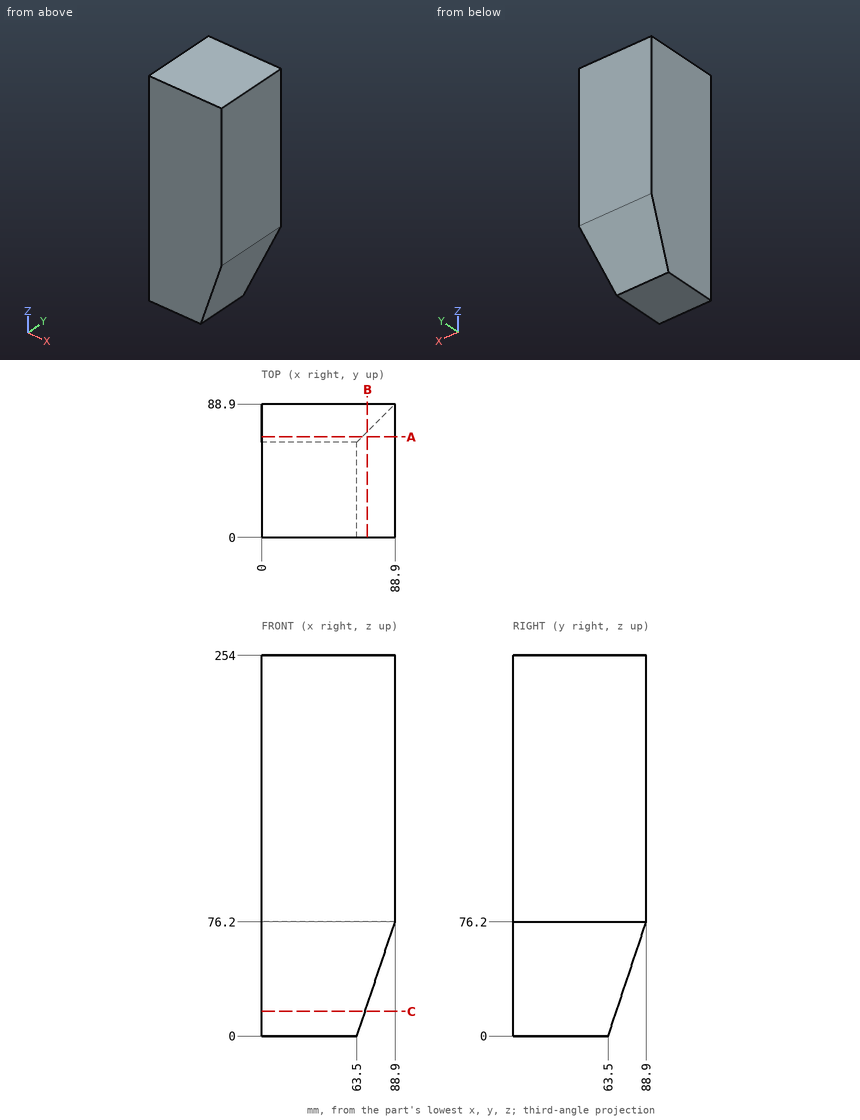
Here's the drawing with two shaded views (mm, measured from the low corner). I have some questions. Coordinates: 2 decimals unless noted, no trailing zeros. Loops run counter-clockwise (first coordinate to the right, second up) from the corner with the lowest first, then second, coordinate; pieces in that order, holes last. Notation, with made-up numbers: M -33,-34 L 4,-34 A19 ccw 4,-30 Z; hole C 86.25,-28.5 d2. An arc over 180 degrees is marked long. Put each result on its own line as item: value. Start each with the question number.
(1) Imagine slicing it at B-B on x = 70.5. List the corners of the cut face in (y, z) for me.
(2) I need wall thicknesses on probe 1 along X at (y, z) = (32.5, 61); probe 2 along X at (y, z) = (67.5, 36.5); probe 3 along Y at (x, z) = (66, 34.5). Which ranges of each line are inside material? Lowest first, please.
(3) Imagine slicing it at C-C on z = 16.5. List the corners of the cut face in (x, y) for me, and give its area (3 significant figures).
(4) Imagine slicing it at A-A on y = 67. List the corners of the cut face in (x, z) for me.
Worked answers:
1. outline: M 0,21 L 70.5,21 L 88.9,76.2 L 88.9,254 L 0,254 Z
2. probe 1: x = 0 to 83.83
2. probe 2: x = 0 to 75.67
2. probe 3: y = 0 to 75
3. outline: M 0,0 L 69,0 L 69,69 L 0,69 Z
3. area: 4,760 mm2
4. outline: M 0,10.5 L 67,10.5 L 88.9,76.2 L 88.9,254 L 0,254 Z
